```python
from build123d import *

# Parameters (mm, degrees)
SKETCH2_R               = 2
SKETCH2_W               = 20.1
SKETCH2_H               = 40.1
BOSS_EXTRUDE1_DEPTH     = 3.175
CUT_EXTRUDE1_DEPTH      = 122.340185532
CUT_EXTRUDE1_DEPTH_BACK = 122.340185532
SKETCH3_R               = 1.6
SKETCH4_W               = 7
SKETCH4_H               = 5
CUT_EXTRUDE2_DEPTH      = 3.175


with BuildPart() as part:
    # Sketch2 → Boss-Extrude1 (new body)
    with BuildSketch(Plane(origin=(0, 0, 0), x_dir=(1, 0, 0), z_dir=(0, 1, 0))):
        with BuildLine():
            Line((-13, 0), (-13, -61.6))
            Line((-13, -61.6), (-4, -116.6))
            ThreePointArc((-4, -116.6), (0, -120.6), (4, -116.6))
            Line((4, -116.6), (13, -61.6))
            Line((13, -61.6), (13, 0))
            ThreePointArc((13, 0), (0, 13), (-13, 0))
        make_face()
        with Locations(Location((-5, 4.5, 0), (0, 0, 270))):
            Circle(SKETCH2_R, mode=Mode.SUBTRACT)
        with Locations(Location((-5, -45.6, 0), (0, 0, 270))):
            Circle(SKETCH2_R, mode=Mode.SUBTRACT)
        with Locations(Location((5, -45.6, 0), (0, 0, 90))):
            Circle(SKETCH2_R, mode=Mode.SUBTRACT)
        with Locations(Location((5, 4.5, 0), (0, 0, 90))):
            Circle(SKETCH2_R, mode=Mode.SUBTRACT)
        with Locations((0, -20.55)):
            Rectangle(SKETCH2_W, SKETCH2_H, mode=Mode.SUBTRACT)
    extrude(amount=BOSS_EXTRUDE1_DEPTH)

    # Sketch3 → Cut-Extrude1 (cut, two sides: drawn at the far end of the back side and taken through both)
    with BuildSketch(Plane(origin=(0, 3.175, 0), x_dir=(1, 0, 0), z_dir=(0, 1, 0)).offset(-CUT_EXTRUDE1_DEPTH_BACK)):
        with Locations(Location((10, -59.4, 0), (0, 0, 270))):
            Circle(SKETCH3_R)
        with Locations(Location((10, -51.9, 0), (0, 0, 270))):
            Circle(SKETCH3_R)
        with Locations(Location((-10, -59.4, 0), (0, 0, 270))):
            Circle(SKETCH3_R)
        with Locations(Location((-10, -51.9, 0), (0, 0, 270))):
            Circle(SKETCH3_R)
    extrude(amount=CUT_EXTRUDE1_DEPTH + CUT_EXTRUDE1_DEPTH_BACK, mode=Mode.SUBTRACT)

    # Sketch4 → Cut-Extrude2 (cut)
    with BuildSketch(Plane(origin=(0, 3.175, 0), x_dir=(1, 0, 0), z_dir=(0, 1, 0))):
        with Locations((0, 2)):
            Rectangle(SKETCH4_W, SKETCH4_H)
    extrude(amount=-CUT_EXTRUDE2_DEPTH, mode=Mode.SUBTRACT)


solid = part.part
```
Design review of the part built by this model. Coordinates are the model's own, in mm. A direction names the side the tool comes from. Give positions to 0.01 mm unless a question says otherwise; leave off trailing zeros. Write each loop counter-clockwise with the first axis right and the second up, starting at its lowest first coordinate (ties: lowest second). Pieces come first, ordered by that corner, then holes. Notation, with made-up numbers: (8.5, 21) - (33.5, 21) arc R27 ccw to (33.5, 39) - close; hole circle Ø6 at (-25.5, 48). An arc over 180 degrees is marked (long way). Return JSON: item names as keys, results as strings. Group by question number.
(1) Mouldability with a two-part tool opening along Z and no side actions: class faces 1 (the flat face through (0, 0, 53)), 2 (the cylindrical face through (-0.1, 1.6, 120.6)), 3 (the flat face through (-10.05, 2, 21)) as +Z half, -Z half, draft (parallel to the pull), parting line (faces both ways), or undercut.
(2) We need section A-A, the plane z = 38.5. Give the boundary of the cut face in (x, y) (3 decimals), then the cut area to 3 significant figures.
(3) Insertion check: pin 1 (1.5 mm diameter, centred on x = 6.5, y = 1, fed in from -Z); pin 2 (8 mm diameter, centred on x = 7, z = 88, fed in from -Y); pin 3 (3 mm diameter, centred on x = 10, z = 51.9, fed in from +Y); pin 4 (1 mm diameter, centred on x = -3, y = 1.5, fed in from -Z). Each pin has a flat end and moves straight along its axis. Give the tip position at first contact, or say it passes through.
(4) We need section D-D, the plane x = 0. Give the boundary of the cut face in (y, z) (3 decimals), then the cut area to 3 significant figures.
(5) To check wall thickness, follow probe 1 along X at (y, z) = (0.8, 45.6); probe 2 along X at (y, z) = (1.5, 51.9); probe 3 along X at (y, z) = (0.6, 12). State the ranges of each line that lie inside material, in increasing order.
(6) Machinability: for faces 4 (the flat face through (-8.563, 1.565, 88.715)), 5 (the flat face through (0, 2, -4.5)), which of the approach directions +Z, -Z, +X, -X, +Y, -Y give a long, thin tool a straight path to every point of the face, cutting with its end or side? Answer none if there is none.
(7) We need section C-C, the plane z = 51.9. Give the boundary of the cut face in (x, y) (3 decimals).
(8) We need section B-B, the plane y = 1.5. Give the boundary of the cut face in (x, z).
Reported:
{
 "1": {"face 1": "draft", "face 2": "+Z half", "face 3": "undercut"},
 "2": {"outline": "(-13, 0) - (-10.05, 0) - (-10.05, 3.175) - (-13, 3.175) - close; (10.05, 0) - (13, 0) - (13, 3.175) - (10.05, 3.175) - close", "area": "18.7 mm2"},
 "3": {"pin 1": "stops at z = -11.66", "pin 2": "stops at y = 0", "pin 3": "passes through", "pin 4": "stops at z = -12.76"},
 "4": {"outline": "(0, -13) - (3.175, -13) - (3.175, -4.5) - (0, -4.5) - close; (0, 40.6) - (3.175, 40.6) - (3.175, 120.6) - (0, 120.6) - close", "area": "281 mm2"},
 "5": {"probe 1": "x = -13 to -7, -3 to 3, 7 to 13", "probe 2": "x = -13 to -11.6, -8.4 to 8.4, 11.6 to 13", "probe 3": "x = -13 to -10.05, 10.05 to 13"},
 "6": {"face 4": "+Z, -X, +Y, -Y", "face 5": "+Y, -Y"},
 "7": {"outline": "(-13, 0) - (-11.6, 0) - (-11.6, 3.175) - (-13, 3.175) - close; (-8.4, 0) - (8.4, 0) - (8.4, 3.175) - (-8.4, 3.175) - close; (11.6, 0) - (13, 0) - (13, 3.175) - (11.6, 3.175) - close"},
 "8": {"outline": "(-13, 0) arc R13 ccw to (13, 0) - (13, 61.6) - (4, 116.6) arc R4 ccw to (-4, 116.6) - (-13, 61.6) - close; hole circle Ø3.2 at (-10, 51.9); hole circle Ø3.2 at (-10, 59.4); hole (-10.05, 0.5) - (-3.5, 0.5) - (-3.5, -3.18) arc R2 ccw (long way) to (-3, -4.5) - (3, -4.5) arc R2 ccw (long way) to (3.5, -3.18) - (3.5, 0.5) - (10.05, 0.5) - (10.05, 40.6) - (-10.05, 40.6) - close; hole circle Ø4 at (-5, 45.6); hole circle Ø4 at (5, 45.6); hole circle Ø3.2 at (10, 51.9); hole circle Ø3.2 at (10, 59.4)"}
}
